Could you check a few things on this model? Use its own coordinates, in mm. Face numbers are marked on the shaded views. A direction names the side the tool comes from. Coordinates: 2 decimals unless noted, no trailing zeros. Order: outer loops, then holes, each group sorted by start corner. A loop starts at its lowest first (then second) coordinate and runs counter-clockwise, first axis right, second up. Notation, with made-up numbers: M -39,80 L -16,80 A20 ccw -16,107 Z; hole C 35,-34.5 d9. An arc over 180 degrees is marked long. Write item = value, one per line. Start each with the question number.
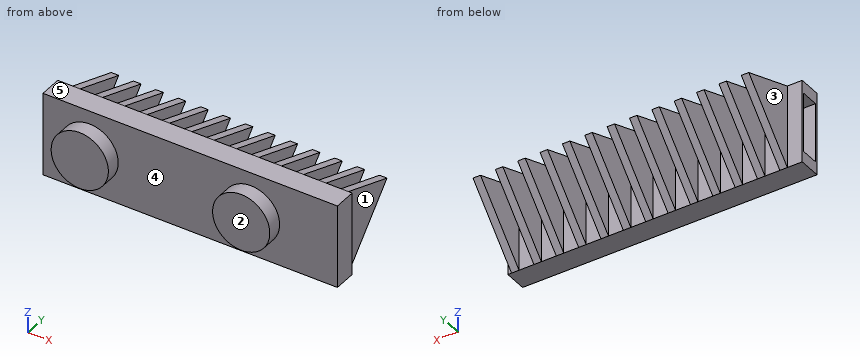
from build123d import *

# Parameters (mm, degrees)
SKETCH1_W           = 211.1375
SKETCH1_H           = 35.56
BOSS_EXTRUDE1_DEPTH = 9.525
SKETCH6_R           = 12.192
BOSS_EXTRUDE4_DEPTH = 6.35
BOSS_EXTRUDE5_DEPTH = 3.175
LPATTERN1_COUNT     = 22
LPATTERN1_PITCH     = 9.525
SKETCH10_W          = 45.550099835
SKETCH10_H          = 62.093170918
CUT_EXTRUDE1_DEPTH  = 85.725
SKETCH11_W          = 25.4
SKETCH11_H          = 7.62
CUT_EXTRUDE2_DEPTH  = 12.7


with BuildPart() as part:
    # Sketch1 → Boss-Extrude1 (new body)
    with BuildSketch(Plane(origin=(0, 0, 0), x_dir=(1, 0, 0), z_dir=(0, 1, 0))):
        with Locations((-105.56875, 17.78)):
            Rectangle(SKETCH1_W, SKETCH1_H)
    extrude(amount=BOSS_EXTRUDE1_DEPTH)

    # Sketch6 → Boss-Extrude4 (add)
    with BuildSketch(Plane(origin=(0, 0, 0), x_dir=(-1, 0, 0), z_dir=(0, -1, 0))):
        with Locations((105.56875, 17.78)):
            Circle(SKETCH6_R)
        with Locations((36.79825, 17.78)):
            Circle(SKETCH6_R)
        with Locations((174.33925, 17.78)):
            Circle(SKETCH6_R)
    extrude(amount=BOSS_EXTRUDE4_DEPTH)

    # Sketch9 → Boss-Extrude5 (add)
    with BuildSketch(Plane.ZY.offset(204.7875)):
        Polygon((-35.56, 9.525), (0, 9.525), (-8.89, 34.417), align=None)
    boss_extrude5 = extrude(amount=-BOSS_EXTRUDE5_DEPTH)

    # LPattern1: Boss-Extrude5 ×22
    with Locations(*[(i * LPATTERN1_PITCH, 0, 0) for i in range(1, LPATTERN1_COUNT)]):
        add(boss_extrude5)

    # Sketch10 → Cut-Extrude1 (cut)
    with BuildSketch(Plane.ZY.offset(211.1375)):
        with Locations((-16.930184705, 4.77052578)):
            Rectangle(SKETCH10_W, SKETCH10_H)
    extrude(amount=-CUT_EXTRUDE1_DEPTH, mode=Mode.SUBTRACT)

    # Sketch11 → Cut-Extrude2 (cut)
    with BuildSketch(Plane.ZY.offset(125.4125)):
        with Locations((-17.78, 4.7625)):
            Rectangle(SKETCH11_W, SKETCH11_H)
    extrude(amount=-CUT_EXTRUDE2_DEPTH, mode=Mode.SUBTRACT)


solid = part.part
(1) Imagine slicing it at C-C on y = 11.5. Give the number of separate pieces and of enclosed holes in the cut face, plus the area to 3 significant figures.
(2) For the marked faces 1 and 2, which set-ups out of +Z, -Z, +X, -X, +Y, -Y let a thin tool reach every point of the face, with its end or its side?
(3) Imagine slicing it at B-B on x = -26.5. List the corners of the cut face in (y, z) for me (3 decimals).
(4) Will these pins go through, and if not, where does the flat tip stop? P1, Ø7.5, axis at y = 19, z = -24, coming from the +X side; P2, Ø3, axis at y = 13.5, z = -6, coming from the -X side; P3, Ø12, axis at x = -96.5, y = 7, coming from the +Z side; P4, Ø7, axis at x = -56.5, z = -23.5, coming from the +Y side.
(5) Thinking about a two-plate mould opening in X: for the marked faces 3, 4 and 5, which applies, released by +X, released by -X, zero draft, split by the parting line, or undercut?
(6) Imagine slicing it at A-A on y = 4. List the corners of the cut face in (x, z) for me.
(7) Please list where these lines run through material, in increasing order: probe 1 along Z at (x, y) = (-114.5, 8); probe 2 along Y at (x, z) = (-119.5, -22.5) (1 decimal); probe 3 along Y at (x, z) = (-75.5, -17) (3 decimals). Write a range as from..to.
Response:
q1.separate_pieces = 13
q1.enclosed_holes = 0
q1.area = 1,350 mm2
q2.face_1 = +Z, -Z, +X, +Y
q2.face_2 = +Z, -Z, +X, -X, -Y
q3.outline = M -6.35,-24.306 L 0,-24.306 L 0,-35.56 L 9.525,-35.56 L 9.525,0 L 0,0 L 0,-11.254 L -6.35,-11.254 Z
q4.P1 = -1.59
q4.P2 = -119.06
q4.P3 = 0
q4.P4 = 23.29
q5.face_3 = released by -X
q5.face_4 = undercut
q5.face_5 = zero draft
q6.outline = M -125.41,-35.56 L 0,-35.56 L 0,0 L -125.41,0 L -125.41,-5.08 L -112.71,-5.08 L -112.71,-30.48 L -125.41,-30.48 Z
q7.probe_1 = -35.56..-30.48, -5.08..0
q7.probe_2 = 0..1, 8.6..9.5
q7.probe_3 = 0..9.525
